Source: CAD feature listing. Evaluate the final solid. Frame: model axes, mm. Face numbers are marked on the shaded views. A direction names the side the tool comes from. Give positions to 0.01 mm unless a question says otherwise; leave off trailing zeros. Order: outer loops, then holes, each group sorted by start corner. A loop starts at its lowest first (then second) coordinate and runs counter-clockwise, first axis right, second up. Notation, with made-up numbers: (-35.5, 28) - (15.5, 28) arc R27 cw to (15.5, 59) - close; hole circle Ø1 at (61.5, 67.25). An arc over 180 degrees is marked (long way). Use CSV: the item, a comma, the result in double quotes.
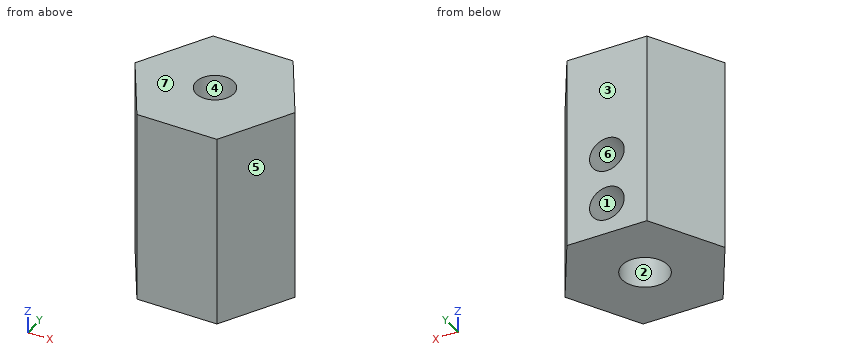
```python
from build123d import *

# Parameters (mm, degrees)
BOSS_EXTRUDE1_DEPTH        = 8.5
CUT_EXTRUDE1_START         = -10
SKETCH2_R                  = 2
CUT_EXTRUDE1_DEPTH         = 10
M4X0_7_TAPPED_HOLE1_D      = 3.3
M4X0_7_TAPPED_HOLE1_DEPTH  = 7
M4X0_7_TAPPED_HOLE1_TIP    = 0.991420021
M3X0_5_TAPPED_HOLE1_REACH  = 18.256
M3X0_5_TAPPED_HOLE1_BORE_R = 1.5


with BuildPart() as part:
    # Sketch1 → Boss-Extrude1 (new, symmetric)
    with BuildSketch(Plane.XY):
        Polygon((3.464101615, 6), (-3.464101615, 6), (-6.92820323, 0), (-3.464101615, -6), (3.464101615, -6), (6.92820323, 0), align=None)
    extrude(amount=BOSS_EXTRUDE1_DEPTH, both=True)

    # Sketch2 → Cut-Extrude1 (cut)
    with BuildSketch(Plane(origin=(0, 0, -8.5), x_dir=(-1, 0, 0), z_dir=(0, 0, -1)).offset(CUT_EXTRUDE1_START)):
        Circle(SKETCH2_R)
    extrude(amount=CUT_EXTRUDE1_DEPTH, mode=Mode.SUBTRACT)

    # M4x0.7 Tapped Hole1
    with Locations(Plane.XY.offset(8.5)):
        with Locations((0, 0)):
            Hole(M4X0_7_TAPPED_HOLE1_D / 2, depth=M4X0_7_TAPPED_HOLE1_DEPTH)
            with Locations((0, 0, -(M4X0_7_TAPPED_HOLE1_DEPTH + M4X0_7_TAPPED_HOLE1_TIP / 2))):  # 118° drill point
                Cone(0, M4X0_7_TAPPED_HOLE1_D / 2, M4X0_7_TAPPED_HOLE1_TIP, mode=Mode.SUBTRACT)

    # M3x0.5 Tapped Hole1 bore → M3x0.5 Tapped Hole1 (cut, up to next)
    with BuildSketch(Plane(origin=(0, 6, 0), x_dir=(1, 0, 0), z_dir=(0, 1, 0)), mode=Mode.PRIVATE) as m3x0_5_tapped_hole1_sk1:
        with Locations((0, 5.75)):
            Circle(M3X0_5_TAPPED_HOLE1_BORE_R)
    m3x0_5_tapped_hole1_tool1 = extrude(m3x0_5_tapped_hole1_sk1.sketch, amount=-M3X0_5_TAPPED_HOLE1_REACH, mode=Mode.PRIVATE) & part.part
    # M3x0.5 Tapped Hole1 bore → M3x0.5 Tapped Hole1 (cut, up to next)
    with BuildSketch(Plane(origin=(0, 6, 0), x_dir=(1, 0, 0), z_dir=(0, 1, 0)), mode=Mode.PRIVATE) as m3x0_5_tapped_hole1_sk2:
        with Locations((0, 1.25)):
            Circle(M3X0_5_TAPPED_HOLE1_BORE_R)
    m3x0_5_tapped_hole1_tool2 = extrude(m3x0_5_tapped_hole1_sk2.sketch, amount=-M3X0_5_TAPPED_HOLE1_REACH, mode=Mode.PRIVATE) & part.part
    add(m3x0_5_tapped_hole1_tool1.solids().sort_by_distance((0, 6, -5.75))[0], mode=Mode.SUBTRACT)
    add(m3x0_5_tapped_hole1_tool2.solids().sort_by_distance((0, 6, -1.25))[0], mode=Mode.SUBTRACT)


solid = part.part
```
Item 1: First-contact query: pin 1 (4.5 mm diameter, centred on x = 0, y = 0, fed in from +Z); pin 2 (6 mm diameter, centred on y = 4.5, z = 0.5, fed in from +X); pin 3 (2.5 mm diameter, centred on x = 0, y = 0, fed in from -Z); pin 4 (2.5 mm diameter, centred on x = 0, z = -5.75, fed in from +Y). Flat tips, straight axial feed; report the tip coordinate or a pass-through.
Filled in:
pin 1,"stops at z = 8.5"
pin 2,"stops at x = 6.06"
pin 3,"passes through"
pin 4,"stops at y = -1.56"
Item 2: Section D-D on z = -5.75. Return the cut outline in (x, y), then the cut area to 3 significant figures.
Filled in:
outline,"(-6.93, 0) - (-3.46, -6) - (3.46, -6) - (6.93, 0) - (3.46, 6) - (1.5, 6) - (1.5, 1.32) arc R2 cw (long way) to (-1.5, 1.32) - (-1.5, 6) - (-3.46, 6) - close"
area,"99.5 mm2"
Item 3: Section A-A on x = 0. Return the cut outline in (y, z), then the cut area to 3 significant figures.
Filled in:
outline,"(-6, -8.5) - (-2, -8.5) - (-2, 1.5) - (-1.65, 1.5) - (-1.65, 8.5) - (-6, 8.5) - close; (1.65, 1.5) - (2, 1.5) - (2, 0.25) - (6, 0.25) - (6, 8.5) - (1.65, 8.5) - close; (2, -8.5) - (6, -8.5) - (6, -7.25) - (2, -7.25) - close; (2, -4.25) - (6, -4.25) - (6, -2.75) - (2, -2.75) - close"
area,"117 mm2"
Item 4: Set-up query: the marked faces 1, 2 and 3. Return all of +Z, -Z, +X, -X, +Y, -Y with unobstructed straight access to the full face (end or side cutting, diameter ignored); none if empty.
Filled in:
face 1,"+Y"
face 2,"-Z"
face 3,"+Z, -Z, +X, -X, +Y"
Item 5: Material intervals for line 1 (Z direction, x = 0, y = 3.65); line 2 (Y direction, x = 0, z = 6.75); line 3 (Y direction, x = 0, z = -6.25), sorted ascending. Write a range as from..to.
Filled in:
line 1,"z = -8.5..-7.25, -4.25..-2.75, 0.25..8.5"
line 2,"y = -6..-1.65, 1.65..6"
line 3,"y = -6..-2"
Item 6: Mould query, pull axis X, two halves, no side actions, for the marked faces 4, 5, 6 and 7. Classes: released by +X, released by -X, zero draft, split by the parting line, or undercut.
Filled in:
face 4,"undercut"
face 5,"released by +X"
face 6,"undercut"
face 7,"zero draft"
Item 7: Section C-C on z = 4.5. Return the cut outline in (x, y), then the cut area to 3 significant figures.
Filled in:
outline,"(-6.93, 0) - (-3.46, -6) - (3.46, -6) - (6.93, 0) - (3.46, 6) - (-3.46, 6) - close; hole circle Ø3.3 at (0, 0)"
area,"116 mm2"
Item 8: Section B-B on y = -0.5. Return the cut outline in (x, z), then the cut area to 3 significant figures.
Filled in:
outline,"(-6.64, -8.5) - (-1.94, -8.5) - (-1.94, 1.5) - (-1.57, 1.5) - (-1.57, 8.5) - (-6.64, 8.5) - close; (1.57, 1.5) - (1.94, 1.5) - (1.94, -8.5) - (6.64, -8.5) - (6.64, 8.5) - (1.57, 8.5) - close"
area,"165 mm2"
